```python
from build123d import *

# Parameters (mm, degrees)
SKETCH_1_R               = 5
EXTRUDE_1_DEPTH          = 12.5
SKETCH_2_R               = 6
EXTRUDE_2_DEPTH          = 22.5
SKETCH_3_R               = 5
EXTRUDE_3_DEPTH          = 12.5
SKETCH_4_W               = 12
SKETCH_4_H               = 35
EXTRUDE_4_DEPTH          = 80
EXTRUDE_5_DEPTH          = 12
EXTRUDE_6_DEPTH          = 10
SKETCH_7_R               = 9.5
CUT_EXTRUDE_1_DEPTH      = 2
SKETCH_8_R               = 6
CUT_EXTRUDE_2_DEPTH      = 166.329973084
EXTRUDE_START            = -10
EXTRUDE_7_DEPTH          = 10
SKETCH_10_R              = 2.5
CUT_EXTRUDE_3_DEPTH      = 10
FILLET_1_R               = 5
FILLET_2_R               = 5
SKETCH_11_R              = 2.5
CUT_EXTRUDE_4_DEPTH      = 10
EXTRUDE_8_DEPTH          = 10
SKETCH_13_R              = 12.5
SKETCH_13_R_2            = 2
CUT_EXTRUDE_5_DEPTH      = 10
PATTERN_CIRCULAR_1_COUNT = 8
SKETCH_14_R              = 2.5
EXTRUDE_9_DEPTH          = 10
SKETCH_15_R              = 2.5
CUT_EXTRUDE_6_DEPTH      = 35
CUT_EXTRUDE_7_DEPTH      = 175.719754648
CUT_EXTRUDE_8_DEPTH      = 1
CUT_EXTRUDE_8_DEPTH_BACK = 162.449682564
SKETCH_18_W              = 84.288718948
SKETCH_18_H              = 107.811152142


with BuildPart() as part:
    # 草图1 → 凸台-拉伸1 (new body)
    with BuildSketch(Plane.XY):
        Circle(SKETCH_1_R)
    extrude(amount=EXTRUDE_1_DEPTH)

    # 草图2 → 凸台-拉伸2 (add)
    with BuildSketch(Plane.XY.offset(12.5)):
        with Locations(Location((0, 0, 0), (0, 0, 180))):
            Circle(SKETCH_2_R)
    extrude_2 = extrude(amount=EXTRUDE_2_DEPTH)

    # 镜向2: 凸台-拉伸2 across plane
    add(extrude_2.mirror(Plane.XY.offset(35)))

    # 草图3 → 凸台-拉伸3 (add)
    with BuildSketch(Plane.XY.offset(57.5)):
        Circle(SKETCH_3_R)
    extrude(amount=EXTRUDE_3_DEPTH)

    # 草图4 → 凸台-拉伸4 (add)
    with BuildSketch(Plane(origin=(0, 0, 0), x_dir=(1, 0, 0), z_dir=(0, 1, 0))):
        with Locations((0, -35)):
            Rectangle(SKETCH_4_W, SKETCH_4_H)
    extrude(amount=EXTRUDE_4_DEPTH)

    # 草图5 → 凸台-拉伸5 (add)
    with BuildSketch(Plane.ZY.offset(6)):
        with BuildLine():
            Line((17.5, 65), (17.5, 80))
            Line((17.5, 80), (13, 80))
            ThreePointArc((13, 80), (5.928932188, 82.928932188), (3, 90))
            Line((3, 90), (3, 130))
            Line((3, 130), (-7, 130))
            Line((-7, 130), (-7, 75))
            ThreePointArc((-7, 75), (-4.071067812, 67.928932188), (3, 65))
            Line((3, 65), (17.5, 65))
        make_face()
        with BuildLine():
            Line((59, 80), (52.5, 80))
            Line((52.5, 80), (52.5, 65))
            Line((52.5, 65), (69, 65))
            ThreePointArc((69, 65), (76.071067812, 67.928932188), (79, 75))
            Line((79, 75), (79, 130))
            Line((79, 130), (69, 130))
            Line((69, 130), (69, 90))
            ThreePointArc((69, 90), (66.071067812, 82.928932188), (59, 80))
        make_face()
    extrude(amount=-EXTRUDE_5_DEPTH)

    # 草图6 → 凸台-拉伸6 (add)
    with BuildSketch(Plane(origin=(0, 0, 69), x_dir=(-1, 0, 0), z_dir=(0, 0, -1))):
        with BuildLine():
            Line((6, 116.252272915), (6, 130))
            Line((6, 130), (-6, 130))
            Line((-6, 130), (-6, 116.252272915))
            ThreePointArc((-6, 116.252272915), (0, 115), (6, 116.252272915))
        make_face()
        with BuildLine():
            Line((-6, 130), (6, 130))
            Line((6, 130), (6, 116.252272915))
            ThreePointArc((6, 116.252272915), (12.549900398, 121.784161637), (15, 130))
            ThreePointArc((15, 130), (-8.215838363, 142.549900398), (-6, 116.252272915))
            Line((-6, 116.252272915), (-6, 130))
        make_face()
    extrude(amount=-EXTRUDE_6_DEPTH)

    # 草图7 → 切除-拉伸1 (cut)
    with BuildSketch(Plane(origin=(0, 0, 69), x_dir=(-1, 0, 0), z_dir=(0, 0, -1))):
        with Locations((0, 130)):
            Circle(SKETCH_7_R)
    extrude(amount=-CUT_EXTRUDE_1_DEPTH, mode=Mode.SUBTRACT)

    # 草图8 → 切除-拉伸2 (cut, through all)
    with BuildSketch(Plane(origin=(0, 0, 71), x_dir=(-1, 0, 0), z_dir=(0, 0, -1))):
        with Locations((0, 130)):
            Circle(SKETCH_8_R)
    extrude(amount=-CUT_EXTRUDE_2_DEPTH, mode=Mode.SUBTRACT)

    # 草图9 → 凸台-拉伸7 (add)
    with BuildSketch(Plane.XY.offset(79).offset(EXTRUDE_START)):
        with BuildLine():
            Line((-15, 155), (-15, 130))
            ThreePointArc((-15, 130), (0, 145), (15, 130))
            Line((15, 130), (15, 155))
            Line((15, 155), (-15, 155))
        make_face()
    extrude(amount=EXTRUDE_7_DEPTH)

    # 草图10 → 切除-拉伸3 (cut)
    with BuildSketch(Plane.XY.offset(79)):
        with Locations((10, 150)):
            Circle(SKETCH_10_R)
    extrude(amount=-CUT_EXTRUDE_3_DEPTH, mode=Mode.SUBTRACT)

    # 圆角1
    fillet_1_edges = [part.edges().sort_by_distance(p)[0] for p in [
        (15, 155, 74),
    ]]
    fillet(fillet_1_edges, radius=FILLET_1_R)

    # 圆角2
    fillet_2_edges = [part.edges().sort_by_distance(p)[0] for p in [
        (-15, 155, 74),
    ]]
    fillet(fillet_2_edges, radius=FILLET_2_R)

    # 草图11 → 切除-拉伸4 (cut)
    with BuildSketch(Plane.XY.offset(79)):
        with Locations((-10, 150)):
            Circle(SKETCH_11_R)
    extrude(amount=-CUT_EXTRUDE_4_DEPTH, mode=Mode.SUBTRACT)

    # 草图12 → 凸台-拉伸8 (add)
    with BuildSketch(Plane.XY.offset(3)):
        with BuildLine():
            ThreePointArc((-6, 103.162526199), (0, 102.5), (6, 103.162526199))
            Line((6, 103.162526199), (6, 130))
            Line((6, 130), (-6, 130))
            Line((-6, 130), (-6, 103.162526199))
        make_face()
        with BuildLine():
            Line((6, 130), (6, 103.162526199))
            ThreePointArc((6, 103.162526199), (21.462176031, 112.806251136), (27.5, 130))
            ThreePointArc((27.5, 130), (-17.193748864, 151.462176031), (-6, 103.162526199))
            Line((-6, 103.162526199), (-6, 130))
            Line((-6, 130), (6, 130))
        make_face()
    extrude(amount=-EXTRUDE_8_DEPTH)

    # 草图13 → 切除-拉伸5 (cut)
    with BuildSketch(Plane(origin=(0, 0, -7), x_dir=(-1, 0, 0), z_dir=(0, 0, -1))):
        with Locations(Location((0, 130, 0), (0, 0, 90))):
            Circle(SKETCH_13_R)
        with Locations(Location((0, 150, 0), (0, 0, 90))):
            Circle(SKETCH_13_R_2)
    cut_extrude_5 = extrude(amount=-CUT_EXTRUDE_5_DEPTH, mode=Mode.SUBTRACT)

    # 阵列(圆周)1: 切除-拉伸5 ×8 about axis
    pattern_circular_1_axis = Axis((0, 130, 0), (0, 0, 1))
    for i in range(1, PATTERN_CIRCULAR_1_COUNT):
        add(cut_extrude_5.rotate(pattern_circular_1_axis, i * 360 / PATTERN_CIRCULAR_1_COUNT), mode=Mode.SUBTRACT)

    # 草图14 → 凸台-拉伸9 (add)
    with BuildSketch(Plane(origin=(0, 0, -7), x_dir=(-1, 0, 0), z_dir=(0, 0, -1)).offset(EXTRUDE_START)):
        with BuildLine():
            Line((-6, 161.837473801), (-6, 156.837473801))
            ThreePointArc((-6, 156.837473801), (0, 157.5), (6, 156.837473801))
            Line((6, 156.837473801), (6, 161.837473801))
            ThreePointArc((6, 161.837473801), (4.535533906, 165.373007707), (1, 166.837473801))
            Line((1, 166.837473801), (-1, 166.837473801))
            ThreePointArc((-1, 166.837473801), (-4.535533906, 165.373007707), (-6, 161.837473801))
        make_face()
        with Locations(Location((0, 161.837473801, 0), (0, 0, 90))):
            Circle(SKETCH_14_R, mode=Mode.SUBTRACT)
    extrude(amount=EXTRUDE_9_DEPTH)

    # 草图15 → 切除-拉伸6 (cut)
    with BuildSketch(Plane(origin=(0, 0, 17.5), x_dir=(-1, 0, 0), z_dir=(0, 0, -1))):
        with Locations((0, 25)):
            Circle(SKETCH_15_R)
        with Locations((0, 50)):
            Circle(SKETCH_15_R)
    extrude(amount=-CUT_EXTRUDE_6_DEPTH, mode=Mode.SUBTRACT)

    # 草图16 → 切除-拉伸7 (cut, through all)
    with BuildSketch(Plane.XY.offset(35)):
        Polygon((-6, 97.653254631), (-6, 65), (-6, 15), (6, 15), (6, 65), (6, 97.653254631), align=None)
    extrude(amount=-CUT_EXTRUDE_7_DEPTH, mode=Mode.SUBTRACT)


with BuildPart() as cut_extrude_7_kept_piece:
    # of the separate pieces the step leaves, the one the design keeps (cut_extrude_7_pieces_kept)
    add(part.part.solids().sort_by_distance((-10, 155, 69))[0])

    # 草图18 → 切除-拉伸8 (cut, two sides: drawn at the far end of the back side and taken through both)
    with BuildSketch(Plane(origin=(0, 15, 0), x_dir=(1, 0, 0), z_dir=(0, 1, 0)).offset(-CUT_EXTRUDE_8_DEPTH_BACK)):
        with Locations((0, -29.971236553)):
            Rectangle(SKETCH_18_W, SKETCH_18_H)
    extrude(amount=CUT_EXTRUDE_8_DEPTH + CUT_EXTRUDE_8_DEPTH_BACK, mode=Mode.SUBTRACT)


solid = cut_extrude_7_kept_piece.part
```
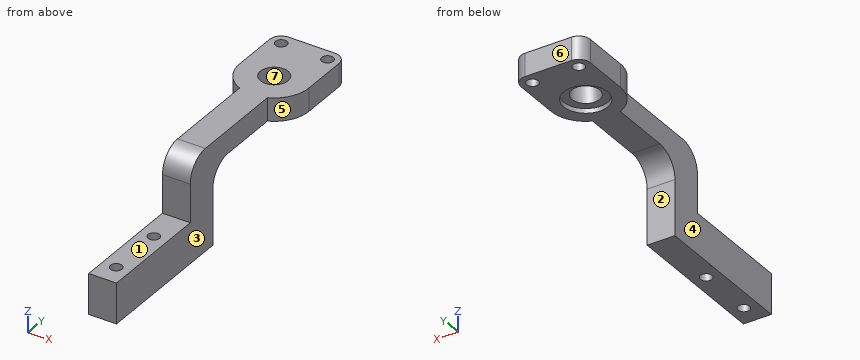
The model under review builds one solid part; all positions refer to its coordinate system, in mm. Face numbers are marked on the shaded views. A direction names the side the tool comes from. Give positions to 0.01 mm unless a question says otherwise; leave off trailing zeros. Write each loop counter-clockwise with the first axis right and the second up, starting at its lowest first coordinate (ties: lowest second). Pieces come first, ordered by that corner, then holes. Notation, with made-up numbers: M 42.5,15 L 92.5,15 A11 cw 92.5,34 Z; hole C -23.5,-8 d7. An arc over 180 degrees is marked long. Answer in a Markdown table with one row per item.
Item 1: Add section B-B on x = 0. Give the boundary of the cut face in (y, z).
Check sheet entries:
| item | result |
|---|---|
| outline | M 16,35 L 22.5,35 L 22.5,52.5 L 16,52.5 Z; M 27.5,35 L 47.5,35 L 47.5,52.5 L 27.5,52.5 Z; M 52.5,35 L 80,35 L 80,59 A10 cw 90,69 L 120.5,69 L 120.5,71 L 124,71 L 124,79 L 75,79 A10 ccw 65,69 L 65,52.5 L 52.5,52.5 Z; M 136,71 L 139.5,71 L 139.5,69 L 155,69 L 155,79 L 136,79 Z |
Item 2: Add section D-D on y = 67. Give the boundary of the cut face in (x, z), plus the area to 3 significant figures.
Check sheet entries:
| item | result |
|---|---|
| outline | M -6,35 L 6,35 L 6,75 L -6,75 Z |
| area | 480 mm2 |
Item 3: Add section C-C on z = 43. Give the boundary of the cut face in (x, y), plus the area to 3 significant figures.
Check sheet entries:
| item | result |
|---|---|
| outline | M -6,16 L 6,16 L 6,80 L -6,80 Z; hole C 0,25 d5; hole C 0,50 d5 |
| area | 729 mm2 |
Item 4: Tool access review of the marked faces 1, 2, 3 and 4: name each direction out of +Z, -Z, +X, -X, +Y, -Y from which nothing blocks a thin tool from reaching the whole face with its end or side.
Check sheet entries:
| item | result |
|---|---|
| face 1 | +Z, +X, -X, -Y |
| face 2 | -Z, +X, -X, +Y |
| face 3 | +Z, -Z, +X, -Y |
| face 4 | +Z, -Z, -X, -Y |
Item 5: For P1, Ø3, axis at x = -1.5, z = 70.5, coming from the -Y side; P2, Ø4, axis at x = -5, z = 58, coming from the +Y side; P3, Ø10, axis at y = 45, z = 40, coming from the +X side; P4, Ø4.5, axis at x = 0, y = 50, coming from the -Z side, all flat-tipped, find the tip position at first contact; note any pin that passes through.
Check sheet entries:
| item | result |
|---|---|
| P1 | y = 65 |
| P2 | y = 80.05 |
| P3 | x = 6 |
| P4 | through |
Item 6: For line 1 along X through (y, z) = (150, 72.5); line 2 along Y through (x, z) = (0, 45); line 3 along Z through (x, y) = (-9.5, 120.5), list the stretches that pass through material, from the lowest coordinate up.
Check sheet entries:
| item | result |
|---|---|
| line 1 | -15 to -12.5, -7.5 to 7.5, 12.5 to 15 |
| line 2 | 16 to 22.5, 27.5 to 47.5, 52.5 to 80 |
| line 3 | 69 to 79 |
Item 7: Draft analysis for pull direction X (two halves, no side actions). For the marked faces 5, 6 and 7, state which applies: +X half, -X half, draft (parallel to the pull), parting line (faces both ways), or undercut.
Check sheet entries:
| item | result |
|---|---|
| face 5 | +X half |
| face 6 | draft |
| face 7 | undercut |
Item 8: Add section A-A on y = 25. Give the boundary of the cut face in (x, z).
Check sheet entries:
| item | result |
|---|---|
| outline | M -6,35 L -2.5,35 L -2.5,52.5 L -6,52.5 Z; M 2.5,35 L 6,35 L 6,52.5 L 2.5,52.5 Z |
